Can you work these out from the model? Positions are in its coordinate system, mm. Give positions to 0.01 mm unless a question says otherwise; leave off trailing zeros. Write each loop counter-clockwise with the first axis right and the second up, starting at its lowest first coordinate (ties: lowest second). Pieces come first, ordered by that corner, then holes. Notation, with made-up numbers: (69, 5.25) -> (116, 5.25) arc R10 ccw to (116, 14.25) -> close; hole circle Ø1 at (89.25, 73.25). An arc over 180 degrees is marked (long way). One line per item, written item: value.
from build123d import *

# Parameters (mm, degrees)
BOSS_EXTRUDE1_DEPTH = 6.35
SKETCH3_R           = 3.302
CUT_EXTRUDE2_DEPTH  = 6.35
SKETCH4_R           = 5.588
CUT_EXTRUDE3_DEPTH  = 2.54
CHAMFER1_SIZE       = 1.016


with BuildPart() as part:
    # Sketch1 → Boss-Extrude1 (new body)
    with BuildSketch(Plane(origin=(0, 0, 0), x_dir=(1, 0, 0), z_dir=(0, 1, 0))):
        Polygon((-7.240727314, -173.10442994), (68.959272686, -173.10442994), (68.959272686, -96.90442994), (30.859272686, -96.90442994), (30.859272686, -135.00442994), (-7.240727314, -135.00442994), align=None)
    extrude(amount=BOSS_EXTRUDE1_DEPTH)

    # Sketch3 → Cut-Extrude2 (cut)
    with BuildSketch(Plane(origin=(0, 0, 0), x_dir=(1, 0, 0), z_dir=(0, 1, 0))):
        with Locations((11.809272686, -154.05442994)):
            Circle(SKETCH3_R)
        with Locations((49.909272686, -115.95442994)):
            Circle(SKETCH3_R)
    extrude(amount=CUT_EXTRUDE2_DEPTH, mode=Mode.SUBTRACT)

    # Sketch4 → Cut-Extrude3 (cut)
    with BuildSketch(Plane(origin=(0, 6.35, 0), x_dir=(1, 0, 0), z_dir=(0, 1, 0))):
        with Locations((11.809272686, -154.05442994)):
            Circle(SKETCH4_R)
        with Locations((49.909272686, -115.95442994)):
            Circle(SKETCH4_R)
    extrude(amount=-CUT_EXTRUDE3_DEPTH, mode=Mode.SUBTRACT)

    # Chamfer1
    chamfer1_edges = [part.edges().sort_by_distance(p)[0] for p in [
        (11.809272686, 6.35, 135.00442994),
        (-7.240727314, 6.35, 154.05442994),
        (30.859272686, 6.35, 173.10442994),
        (68.959272686, 6.35, 135.00442994),
        (49.909272686, 6.35, 96.90442994),
        (30.859272686, 6.35, 115.95442994),
    ]]
    chamfer(chamfer1_edges, length=CHAMFER1_SIZE)


solid = part.part
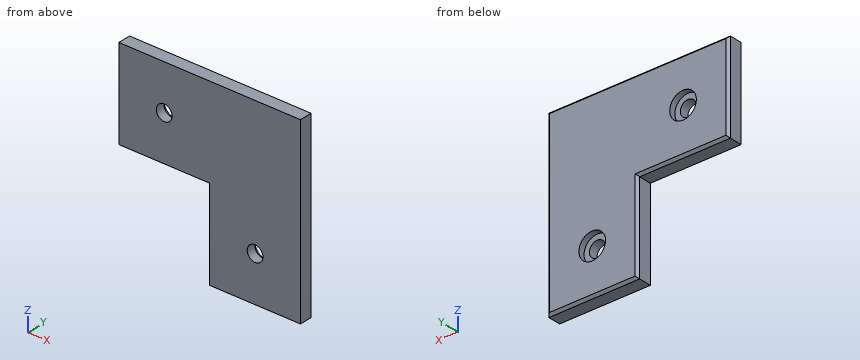
1) I need wall thicknesses on L1, parallel to X at y = 3.25, z = 102; L2, parallel to Z at x = 26.5, y = 1.75; L3, parallel to Y at x = 17, z = 156. Which ranges of each line are inside material? Lowest first, please.
Answer list:
L1: x = 30.86 to 68.96
L2: z = 135 to 173.1
L3: y = 0 to 3.81
2) If we section it at B-B (x = 20): Write out the boundary of the cut face in (y, z), and give its area (3 significant figures).
Answer list:
outline: (0, 135) -> (5.33, 135) -> (6.35, 136.02) -> (6.35, 172.09) -> (5.33, 173.1) -> (0, 173.1) -> close
area: 241 mm^2
3) Will these pins go through, and if not, where does the flat tip stop? pin 1 (5.5 mm diameter, centred on x = 52.5, z = 117, fed in from +Y); pin 2 (6.5 mm diameter, centred on x = 49.91, z = 115.95, fed in from -Y); pin 3 (2.5 mm diameter, centred on y = 3, z = 112, fed in from -X); pin 4 (2.5 mm diameter, centred on x = 6, y = 3, fed in from -Z).
Answer list:
pin 1: stops at y = 3.81
pin 2: passes through
pin 3: stops at x = 30.86
pin 4: stops at z = 135
4) If we section it at C-C (x = 12): Write out the boundary of the cut face in (y, z).
Answer list:
outline: (0, 135) -> (5.33, 135) -> (6.35, 136.02) -> (6.35, 148.47) -> (3.81, 148.47) -> (3.81, 150.76) -> (0, 150.76) -> close; (0, 157.35) -> (3.81, 157.35) -> (3.81, 159.64) -> (6.35, 159.64) -> (6.35, 172.09) -> (5.33, 173.1) -> (0, 173.1) -> close
5) If we section it at A-A (z = 117.5): Write out the boundary of the cut face in (x, y).
Answer list:
outline: (30.86, 0) -> (46.99, 0) -> (46.99, 3.81) -> (44.54, 3.81) -> (44.54, 6.35) -> (31.88, 6.35) -> (30.86, 5.33) -> close; (52.83, 0) -> (68.96, 0) -> (68.96, 5.33) -> (67.94, 6.35) -> (55.28, 6.35) -> (55.28, 3.81) -> (52.83, 3.81) -> close
